```python
from build123d import *

# Parameters (mm, degrees)
F1_DEPTH = 50
F2_W     = 3
F2_H     = 50
F3_DEPTH = 15
F4_W     = 3
F4_H     = 50
F5_DEPTH = 15
F9_DEPTH = 50


with BuildPart() as f1:
    # F0 (on Top) → F1 (new body)
    with BuildSketch(Plane.XY):
        with BuildLine():
            Line((0, 13.42), (8.94, 13.42))
            ThreePointArc((8.94, 13.42), (15.665114, 0.270758), (10.125, -13.42))
            Line((10.125, -13.42), (0, -13.42))
            Line((0, -13.42), (0, -16.42))
            Line((0, -16.42), (11.265835, -16.42))
            ThreePointArc((11.265835, -16.42), (18.665454, 0.325994), (9.93816, 16.42))
            Line((9.93816, 16.42), (0, 16.42))
            Line((0, 16.42), (0, 13.42))
        make_face()
    extrude(amount=F1_DEPTH)

    # F2 (on face) → F3 (join)
    with BuildSketch(Plane(origin=(0, 0, 0), x_dir=(0, -1, 0), z_dir=(-1, 0, 0))):
        with Locations((-14.92, 25)):
            Rectangle(F2_W, F2_H)
    extrude(amount=F3_DEPTH)

    # F4 (on face) → F5 (join)
    with BuildSketch(Plane(origin=(0, 0, 0), x_dir=(0, -1, 0), z_dir=(-1, 0, 0))):
        with Locations((14.92, 25)):
            Rectangle(F4_W, F4_H)
    extrude(amount=F5_DEPTH)

    # F8 (on Top) → F9 (join)
    with BuildSketch(Plane.XY):
        with BuildLine():
            Line((-12, 13.42), (-15, 13.42))
            ThreePointArc((-15, 13.42), (-13.5, 11.744685), (-12, 13.42))
        make_face()
    extrude(amount=F9_DEPTH)


solid = f1.part
```
The model under review builds one solid part; all positions refer to its coordinate system, in mm. A direction names the side the tool comes from. Give positions to 0.01 mm unless a question says otherwise; leave off trailing zeros. Write each loop counter-clockwise with the first axis right and the second up, starting at its lowest first coordinate (ties: lowest second). Pieces come first, ordered by that corner, then holes.
(1) Consider section C-C, the plane x = 7. Give the boundary of the cut face in (y, z), and give its area (3 significant figures).
(2) Consider section D-D, the plane y = -12.5. Give the boundary of the cut face in (x, z), and give its area (3 significant figures).
(3) The part is to be moulded in two halves that separate along Y. For faces 4 (the flat face through (-15, -15, 25)), 5 (the cylindrical face through (-13.536, 11.745, 24.65)), 6 (the cylindrical face through (18.674, 0.061, 24.65)), 7 (the cylindrical face through (15.654, 0.484, 24.65)), say which applies: released by +Y, released by -Y, zero draft, split by the parting line, or undercut.
(4) Consider section A-A, the plane x = -13.5. Give the boundary of the cut face in (y, z).
(5) For P1, Ø1.5, axis at y = -4, z = 42, coming from the +X side; P2, Ø1.5, axis at y = -14, z = 16, coming from the -X side; P3, Ø8, axis at y = 8.5, z = 5, coming from the +X side, all flat-tipped, find the tip position at first contact; note any pin that passes through.
(6) Consider section B-B, the plane z = 32. Give the boundary of the cut face in (x, y) (3 decimals), and give its area (3 significant figures).
(7) Tool access review of faces 1 (the flat face through (-2, -13.42, 25)), 2 (the flat face through (-2, -16.42, 25)), 3 (the flat face through (-1, 13.42, 25)): name each direction out of +Z, -Z, +X, -X, +Y, -Y from which nothing blocks a thin tool from reaching the whole face with its end or side.
(8) To check wall thickness, follow L1, parallel to Y at x = -11, z = 30; L2, parallel to Y at x = 13.5, z = 20; L3, parallel to X at y = 3, z = 13. State the ranges of each line that lie inside material, in increasing order.
Returned:
1. outline: (-16.42, 0) - (-13.42, 0) - (-13.42, 50) - (-16.42, 50) - close; (13.42, 0) - (16.42, 0) - (16.42, 50) - (13.42, 50) - close
1. area: 300 mm2
2. outline: (11.03, 0) - (14.87, 0) - (14.87, 50) - (11.03, 50) - close
2. area: 192 mm2
3. face 4: zero draft
3. face 5: undercut
3. face 6: split by the parting line
3. face 7: undercut
4. outline: (-16.42, 0) - (-13.42, 0) - (-13.42, 50) - (-16.42, 50) - close; (11.74, 0) - (16.42, 0) - (16.42, 50) - (11.74, 50) - close
5. P1: stops at x = 18.5
5. P2: stops at x = -15
5. P3: stops at x = 18.07
6. outline: (-15, -16.42) - (11.266, -16.42) arc R20.767 ccw to (9.938, 16.42) - (-15, 16.42) - (-15, 13.42) arc R1.509 ccw (long way) to (-12, 13.42) - (8.94, 13.42) arc R17.767 cw to (10.125, -13.42) - (-15, -13.42) - close
6. area: 257 mm2
7. face 1: +Z, -Z, -X
7. face 2: +Z, -Z, +X, -X, -Y
7. face 3: +Z, -Z
8. L1: y = -16.42 to -13.42, 13.42 to 16.42
8. L2: y = -14.24 to -9.04, 8.02 to 13.21
8. L3: x = 15.33 to 18.38
